```python
from build123d import *

# Parameters (mm, degrees)
F0_R     = 12.7
F1_DEPTH = 44.45
F3_DEPTH = 12.7
F4_R     = 5.08
F5_DEPTH = 14.7602579501


with BuildPart() as f1:
    # F0 (on Front) → F1 (new body)
    with BuildSketch(Plane.XZ):
        with BuildLine():
            Line((-31.75, -21.59), (0, -21.59))
            Line((0, -21.59), (31.75, -21.5900009905))
            Line((31.75, -21.5900009905), (31.75, -8.89))
            Line((31.75, -8.89), (12.7, -8.89))
            Line((12.7, -8.89), (12.7, 0))
            Line((12.7, 0), (63.4999997359, 0))
            Line((63.4999997359, 0), (63.4999997359, 12.6999990095))
            Line((63.4999997359, 12.6999990095), (47.6249997359, 12.6999990095))
            Line((47.6249997359, 12.6999990095), (21.0934258346, 52.2501726688))
            ThreePointArc((21.0934258346, 52.2501726688), (2.641e-07, 63.5), (-21.0934255404, 52.2501731075))
            Line((-21.0934255404, 52.2501731075), (-47.6250002641, 12.7))
            Line((-47.6250002641, 12.7), (-63.5000002641, 12.7))
            Line((-63.5000002641, 12.7), (-63.5000002641, 0))
            Line((-63.5000002641, 0), (-12.7, 0))
            Line((-12.7, 0), (-12.7, -8.89))
            Line((-12.7, -8.89), (-31.75, -8.89))
            Line((-31.75, -8.89), (-31.75, -21.59))
        make_face()
        with Locations((0, 38.1)):
            Circle(F0_R, mode=Mode.SUBTRACT)
    extrude(amount=F1_DEPTH)

    # F2 (on face) → F3 (join)
    with BuildSketch(Plane(origin=(0, 0, 0), x_dir=(-1, 0, 0), z_dir=(0, 1, 0))):
        Polygon((-63.4999997359, 63.5), (-63.4999997359, 0), (63.5000002641, 0), (63.5000002641, 12.7), (63.5000002641, 63.5000006603), (-2.641e-07, 63.5), align=None)
    extrude(amount=F3_DEPTH)

    # F4 (on face) → F5 (cut, up to face)
    with BuildSketch(Plane.XY.offset(63.5)):
        with Locations((2.641e-07, -22.225)):
            Circle(F4_R)
    extrude(amount=-F5_DEPTH, mode=Mode.SUBTRACT)


solid = f1.part
```
Verification items for the finished model (mm, model axes). A direction names the side the tool comes from. Coordinates: 2 decimals unless noted, no trailing zeros. Order: outer loops, then holes, each group sorted by start corner. A loop starts at its lowest first (then second) coordinate and runs counter-clockwise, first axis right, second up. Notation, with made-up numbers: (59.25, -33) -> (77.25, -33) arc R32 ccw to (77.25, -3) -> close; hole circle Ø5 at (88.5, 30.25). An arc over 180 degrees is marked (long way). Put each result on its own line as item: value. Start each with the question number.
1) Cross-section at A-A (x = -26.5). Enter the section's corners in (y, z).
2) Tool access check on faces 5 (the flat face through (56, -22, 12.7)), 6 (the flat face through (-31.75, -22, -15)), 7 (the flat face through (-22, -22, -8.89)), 8 (the flat face through (0, 0, -13)). Record the directions out of +Z, -Z, +X, -X, +Y, -Y that give a thin tool (end or side, any length) a straight path to the whole face; none if there is none.
3) Material ranges on L1, parallel to Y at x = -29, z = 53; L2, parallel to X at y = -2, z = -14.5, recorded low to high.
4) Release check for a two-part mould opening along X. For faces 1 (the flat face through (0, 0, 38)), 2 (the flat face through (-45, 0, 44)), 3 (the cylindrical face through (5.86, -21.914, 26.833)), 4 (the flat face through (-34.173, -21.914, 32.752)) record: pulls with the +X half, pulls with the -X half, needs draft (parallel to the pull), parting line crosses it, or undercut.
5) Go/stop test with flat-tipped pins: pin 1 (10 mm diameter, centred on y = -20, z = -6.5, fed in from -X); pin 2 (9.5 mm diameter, centred on x = -25, y = -17.5, fed in from +Z); pin 3 (4 mm diameter, centred on x = 38.5, y = 1.5, fed in from -Z). Record where each tip stops, or that it passes through.
6) Cross-section at C-C (x = 55). Enter the section's corners in (y, z), plus the area to 3 significant figures.
7) Cross-section at D-D (z = 40). Enter the section's corners in (x, y).
8) Cross-section at B-B (y = -31). Enter the section's corners in (x, z) (3 decimals), plus the area to 3 significant figures.
Geometry check:
1. outline: (-44.45, -21.59) -> (0, -21.59) -> (0, -8.89) -> (-44.45, -8.89) -> close; (-44.45, 0) -> (12.7, 0) -> (12.7, 63.5) -> (0, 63.5) -> (0, 44.19) -> (-44.45, 44.19) -> close
2. face 5: +Z, +X, -Y
2. face 6: -Z, -X, +Y, -Y
2. face 7: -X, +Y, -Y
2. face 8: -Z, +X, -X, +Y
3. L1: y = 0 to 12.7
3. L2: x = -31.75 to 31.75
4. face 1: undercut
4. face 2: needs draft
4. face 3: undercut
4. face 4: pulls with the -X half
5. pin 1: stops at x = -31.75
5. pin 2: stops at z = 53.43
5. pin 3: stops at z = 0
6. outline: (-44.45, 0) -> (12.7, 0) -> (12.7, 63.5) -> (0, 63.5) -> (0, 12.7) -> (-44.45, 12.7) -> close
6. area: 1,370 mm^2
7. outline: (-63.5, 0) -> (-29.31, 0) -> (-29.31, -44.45) -> (-12.56, -44.45) -> (-12.56, 0) -> (12.56, 0) -> (12.56, -44.45) -> (29.31, -44.45) -> (29.31, 0) -> (63.5, 0) -> (63.5, 12.7) -> (-63.5, 12.7) -> close
8. outline: (-63.5, 0) -> (-12.7, 0) -> (-12.7, -8.89) -> (-31.75, -8.89) -> (-31.75, -21.59) -> (31.75, -21.59) -> (31.75, -8.89) -> (12.7, -8.89) -> (12.7, 0) -> (63.5, 0) -> (63.5, 12.7) -> (47.625, 12.7) -> (21.093, 52.25) arc R25.4 ccw to (-21.093, 52.25) -> (-47.625, 12.7) -> (-63.5, 12.7) -> close; hole circle Ø25.4 at (0, 38.1)
8. area: 5,190 mm^2
